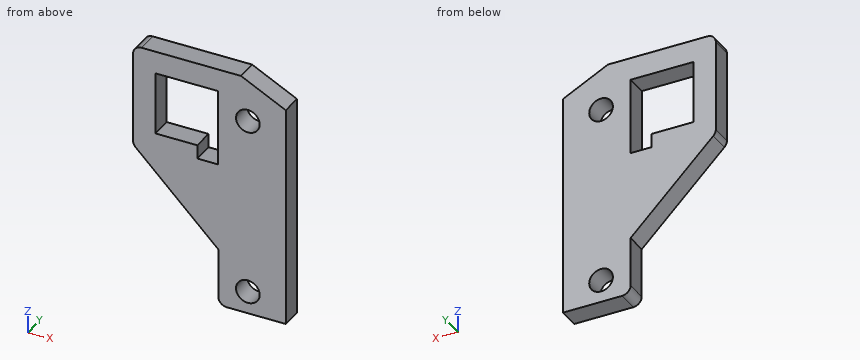
from build123d import *

# Parameters (mm, degrees)
SKETCH1_R           = 1.778
BOSS_EXTRUDE1_DEPTH = 3.175


with BuildPart() as part:
    # Sketch1 → Boss-Extrude1 (new body)
    with BuildSketch(Plane.XZ):
        with BuildLine():
            Line((0, -1.27), (0, -15.096211993))
            ThreePointArc((0, -15.096211993), (0.096672994, -15.582219953), (0.371974388, -15.994237606))
            Line((0.371974388, -15.994237606), (12.811233382, -28.4334966))
            Line((12.811233382, -28.4334966), (12.811233382, -35.9325926))
            ThreePointArc((12.811233382, -35.9325926), (13.18320777, -36.830618212), (14.081233382, -37.2025926))
            Line((14.081233382, -37.2025926), (22.963359382, -37.2025926))
            Line((22.963359382, -37.2025926), (22.963359382, -3.420573773))
            Line((22.963359382, -3.420573773), (16.223955667, 0))
            Line((16.223955667, 0), (1.27, 0))
            ThreePointArc((1.27, 0), (0.371974388, -0.371974388), (0, -1.27))
        make_face()
        with Locations((17.255979382, -33.7812126)):
            Circle(SKETCH1_R, mode=Mode.SUBTRACT)
        with Locations((17.255979382, -6.840444237)):
            Circle(SKETCH1_R, mode=Mode.SUBTRACT)
        Polygon((9.66216, -12.92098), (3.35788, -12.92098), (3.35788, -3.42138), (12.80414, -3.42138), (12.80414, -15.01648), (9.66216, -15.01648), align=None, mode=Mode.SUBTRACT)
    extrude(amount=-BOSS_EXTRUDE1_DEPTH)


solid = part.part
The listing builds one solid part. Answer for the finished solid, in the listing's coordinates (mm). Give positions to 0.01 mm unless a question says otherwise; leave off trailing zeros. Loops run counter-clockwise (first coordinate to the right, second up) from the corner with the lowest first, then second, coordinate; pieces in that order, holes last. Notation, with made-up numbers: (53.25, 24) - (93.25, 24) arc R5 cw to (93.25, 30) - close; hole circle Ø8 at (53, 38.25). An arc over 180 degrees is marked (long way). Answer as a JSON object with one key per item and string values.
1. A cutting plane is placed at C-C (y = 1.05). Write down the section's boundary in (x, z), then the cut area to 3 significant figures.
Determined:
{"outline": "(0, -15.1) arc R1.27 ccw to (0.37, -15.99) - (12.81, -28.43) - (12.81, -35.93) arc R1.27 ccw to (14.08, -37.2) - (22.96, -37.2) - (22.96, -3.42) - (16.22, 0) - (1.27, 0) arc R1.27 ccw to (0, -1.27) - close; hole (3.36, -12.92) - (9.66, -12.92) - (9.66, -15.02) - (12.8, -15.02) - (12.8, -3.42) - (3.36, -3.42) - close; hole circle Ø3.56 at (17.26, -33.78); hole circle Ø3.56 at (17.26, -6.84)", "area": "531 mm²"}
2. A flat-ended cylindrical pin translates along its axis: pin 1 Ø1.5 at (y, z) = (1.5, -18) entering from -X. Find the tip coordinate at first contact, or state that the pin passes through.
Determined:
{"pin 1": "x = 1.63"}
3. A cutting plane is placed at A-A (z = -9.5). Write down the section's boundary in (x, y) (3 decimals).
Determined:
{"outline": "(0, 0) - (3.358, 0) - (3.358, 3.175) - (0, 3.175) - close; (12.804, 0) - (22.963, 0) - (22.963, 3.175) - (12.804, 3.175) - close"}
4. A cutting plane is placed at D-D (z = -5.5). Write down the section's boundary in (x, y) (3 decimals).
Determined:
{"outline": "(0, 0) - (3.358, 0) - (3.358, 3.175) - (0, 3.175) - close; (12.804, 0) - (16.088, 0) - (16.088, 3.175) - (12.804, 3.175) - close; (18.424, 0) - (22.963, 0) - (22.963, 3.175) - (18.424, 3.175) - close"}
5. Find the intervals of material crossed by L1, parallel to X at y = 0.25, z = -10; L2, parallel to Z at x = 10.5, y = 0.25; L3, parallel to X at y = 2.45, z = -16, in increasing order. Write a range as [from, to].
Determined:
{"L1": "[0, 3.36], [12.8, 22.96]", "L2": "[-26.12, -15.02], [-3.42, 0]", "L3": "[0.38, 22.96]"}
6. A cutting plane is placed at B-B (x = 8.25). Write down the section's boundary in (y, z) (3 decimals), then the cut area to 3 significant figures.
Determined:
{"outline": "(0, -23.872) - (3.175, -23.872) - (3.175, -12.921) - (0, -12.921) - close; (0, -3.421) - (3.175, -3.421) - (3.175, 0) - (0, 0) - close", "area": "45.6 mm²"}
